from build123d import *

# Parameters (mm, degrees)
BOSS_EXTRUDE1_DEPTH = 9.5
SKETCH5_R           = 2.38125
CUT_EXTRUDE1_DEPTH  = 1.5
SKETCH9_W           = 21
SKETCH9_H           = 5
BOSS_EXTRUDE6_DEPTH = 9
SKETCH10_W          = 21
SKETCH10_H          = 14
CUT_EXTRUDE4_DEPTH  = 28.626979567
CUT_EXTRUDE5_DEPTH  = 5
SKETCH12_W          = 24
SKETCH12_H          = 9
BOSS_EXTRUDE7_DEPTH = 5
CUT_EXTRUDE6_DEPTH  = 6
SKETCH15_W          = 46
SKETCH15_H          = 3.5
CUT_EXTRUDE7_DEPTH  = 16.5
SKETCH16_W          = 12.5
SKETCH16_H          = 3.5
CUT_EXTRUDE8_DEPTH  = 16.5
BOSS_EXTRUDE8_DEPTH = 5
SKETCH18_W          = 25.5
SKETCH18_H          = 8.5
CUT_EXTRUDE9_DEPTH  = 9
BOSS_EXTRUDE9_DEPTH = 9
FILLET1_R           = 1
SKETCH20_W          = 10.25
SKETCH20_H          = 10
CUT_EXTRUDE10_DEPTH = 2
SKETCH23_W          = 1.838900381
SKETCH23_H          = 2
CUT_EXTRUDE11_DEPTH = 1.5
CHAMFER1_SIZE       = 1
CHAMFER2_SIZE       = 1


with BuildPart() as part:
    # Sketch2 → Boss-Extrude1 (new, symmetric)
    with BuildSketch(Plane.XY):
        Polygon((-12, 3), (-12, 12), (-23, 12), (-23, 0), (23, 0), (23, 12), (12, 12), (12, 3), align=None)
    extrude(amount=BOSS_EXTRUDE1_DEPTH, both=True)

    # Sketch5 → Cut-Extrude1 (cut)
    with BuildSketch(Plane(origin=(0, 12, 0), x_dir=(1, 0, 0), z_dir=(0, 1, 0))):
        with Locations(Location((-19, 1.5, 0), (0, 0, 180))):
            Circle(SKETCH5_R)
        with Locations(Location((19, 1.5, 0), (0, 0, 180))):
            Circle(SKETCH5_R)
    extrude(amount=-CUT_EXTRUDE1_DEPTH, mode=Mode.SUBTRACT)

    # Sketch9 → Boss-Extrude6 (add)
    with BuildSketch(Plane.XZ):
        with Locations((0, -7)):
            Rectangle(SKETCH9_W, SKETCH9_H)
    extrude(amount=BOSS_EXTRUDE6_DEPTH)

    # Sketch10 → Cut-Extrude4 (cut, through all)
    with BuildSketch(Plane.XZ):
        with Locations((0, 2.5)):
            Rectangle(SKETCH10_W, SKETCH10_H)
    extrude(amount=-CUT_EXTRUDE4_DEPTH, mode=Mode.SUBTRACT)

    # Sketch11 → Cut-Extrude5 (cut)
    with BuildSketch(Plane.XY.offset(9.5)):
        Polygon((10.5, 3), (10.5, 0), (23, 0), (23, 12), (12, 12), (12, 3), align=None)
        Polygon((-10.5, 0), (-10.5, 3), (-12, 3), (-12, 12), (-23, 12), (-23, 0), align=None)
    extrude(amount=-CUT_EXTRUDE5_DEPTH, mode=Mode.SUBTRACT)

    # Sketch12 → Boss-Extrude7 (add)
    with BuildSketch(Plane(origin=(0, 0, -9.5), x_dir=(-1, 0, 0), z_dir=(0, 0, -1))):
        with Locations((0, 7.5)):
            Rectangle(SKETCH12_W, SKETCH12_H)
    extrude(amount=-BOSS_EXTRUDE7_DEPTH)

    # Sketch13 → Cut-Extrude6 (cut)
    with BuildSketch(Plane.XY.offset(-4.5)):
        Polygon((-9, 12), (0, 1.274217667), (9, 12), align=None)
    extrude(amount=-CUT_EXTRUDE6_DEPTH, mode=Mode.SUBTRACT)

    # Sketch15 → Cut-Extrude7 (cut)
    with BuildSketch(Plane.XY.offset(-4.5)):
        with Locations((0, 1.75)):
            Rectangle(SKETCH15_W, SKETCH15_H)
    extrude(amount=CUT_EXTRUDE7_DEPTH, mode=Mode.SUBTRACT)

    # Sketch16 → Cut-Extrude8 (cut)
    with BuildSketch(Plane.XY.offset(-4.5)):
        with Locations((-16.75, 1.75)):
            Rectangle(SKETCH16_W, SKETCH16_H)
        with Locations((16.75, 1.75)):
            Rectangle(SKETCH16_W, SKETCH16_H)
    extrude(amount=-CUT_EXTRUDE8_DEPTH, mode=Mode.SUBTRACT)

    # Sketch17 → Boss-Extrude8 (add)
    with BuildSketch(Plane(origin=(0, 0, -9.5), x_dir=(-1, 0, 0), z_dir=(0, 0, -1))):
        Polygon((10.5, 3.5), (23, 3.5), (23, -1.5), (17, -1.5), (17, -6.5), (23, -6.709524617), (23, -9), (10.5, -9), align=None)
    extrude(amount=-BOSS_EXTRUDE8_DEPTH)

    # Sketch18 → Cut-Extrude9 (cut)
    with BuildSketch(Plane.XY.offset(-4.5)):
        with Locations((0, 7.75)):
            Rectangle(SKETCH18_W, SKETCH18_H)
    extrude(amount=CUT_EXTRUDE9_DEPTH, mode=Mode.SUBTRACT)

    # Sketch19 → Boss-Extrude9 (add)
    with BuildSketch(Plane.XY.offset(-4.5)):
        Polygon((-12.75, 3.5), (-23, 3.5), (-23, -1.5), (-17, -1.5), (-17, -6.5), (-23, -6.709524617), (-23, -9), (-12.75, -9), align=None)
    extrude(amount=BOSS_EXTRUDE9_DEPTH)

    # Fillet1
    fillet1_edges = [part.edges().sort_by_distance(p)[0] for p in [
        (-23, -1.5, -2.5),
        (-23, -6.709524617, -2.5),
    ]]
    fillet(fillet1_edges, radius=FILLET1_R)

    # Sketch20 → Cut-Extrude10 (cut)
    with BuildSketch(Plane.XY.offset(4.5)):
        with Locations((-17.875, -4)):
            Rectangle(SKETCH20_W, SKETCH20_H)
    extrude(amount=-CUT_EXTRUDE10_DEPTH, mode=Mode.SUBTRACT)

    # Sketch23 → Cut-Extrude11 (cut)
    with BuildSketch(Plane(origin=(0, 12, 0), x_dir=(1, 0, 0), z_dir=(0, 1, 0))):
        with Locations((-22.080549809, 1.5)):
            Rectangle(SKETCH23_W, SKETCH23_H)
        with Locations((22.080549809, 1.5)):
            Rectangle(SKETCH23_W, SKETCH23_H)
    extrude(amount=-CUT_EXTRUDE11_DEPTH, mode=Mode.SUBTRACT)

    # Chamfer1
    chamfer1_edges = [part.edges().sort_by_distance(p)[0] for p in [
        (-22.080549809, 12, -2.5),
        (22.080549809, 12, -2.5),
    ]]
    chamfer(chamfer1_edges, length=CHAMFER1_SIZE)

    # Chamfer2
    chamfer2_edges = [part.edges().sort_by_distance(p)[0] for p in [
        (16, 12, -9.5),
        (-16, 12, -9.5),
        (4.5, 6.637108833, -9.5),
        (-4.5, 6.637108833, -9.5),
        (23, 7.75, -9.5),
        (16.75, 3.5, -9.5),
        (-23, -8.337606696, -9.5),
        (-17, -4, -9.5),
        (-19.5, -1.5, -9.5),
        (-19.517449748, -6.587911282, -9.5),
        (-22.7193398, -6.980555021, -9.5),
        (-22.707106781, -1.207106781, -9.5),
        (10.5, -2.75, -9.5),
        (-6.25, -9, -9.5),
        (-23, 5.75, -9.5),
    ]]
    chamfer(chamfer2_edges, length=CHAMFER2_SIZE - 0.0001)  # a hair under: the kernel refuses the full size


solid = part.part
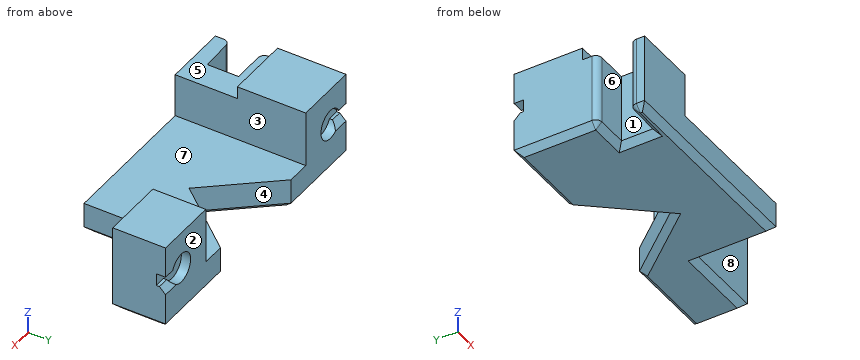
The model under review builds one solid part; all positions refer to its coordinate system, in mm. Face numbers are marked on the shaded views. A direction names the side the tool comes from. Coordinates: 2 decimals unless noted, no trailing zeros. Loops run counter-clockwise (first coordinate to the right, second up) from the corner with the lowest first, then second, coordinate; pieces in that order, holes last. Notation, with made-up numbers: (20, 43.5) -> (74, 43.5) arc R7 ccw to (74, 55.5) -> close; hole circle Ø4 at (49.5, 49.5). An arc over 180 degrees is marked (long way). Use a Markdown table: item, result. Add a question column.
1. To check wall thickness, follow line 1 (Z direction, x = -19, y = 11); line 2 (X direction, y = 11.4, z = -1.5); line 3 (X direction, y = 5.75, z = 1). State the ranges of each line that lie inside material, in increasing order.
2. Add section D-D on z = 3.5. Write out the cut boundary in (x, y), plus the area to 3 significant figures.
3. Add section A-A on z = -1.5. Write out the cut boundary in (x, y).
4. Add section B-B on x = 19. Write out the cut boundary in (y, z), plus the area to 3 significant figures.
5. Draft analysis for pull direction X (two halves, no side actions). For the marked faces 1, 2, 3 and 4, state which applies: pulls with the +X half, pulls with the -X half, needs draft (parallel to the pull), parting line crosses it, or undercut.
6. Add section C-C on y = -3. Write out the cut boundary in (x, z).
7. Machinability: for the marked faces 5, 6, 7 and 8, which of the approach directions +Z, -Z, +X, -X, +Y, -Y give a long, thin tool a straight path to every point of the face, cutting with its end or side? Answer none if there is none.
8. Clearance check with flat-ended pins moving along their axes: pin 1 Ø2.5 at (y, z) = (-5, -1.5) entering from -X; pin 2 Ø8 at (x, y) = (-15.5, -5.5) entering from +Z; pin 3 Ø1 at (x, y) = (6, 6) entering from +Z. State where each tip first meets the part, or that it passes through.
Returned:
| question | item | result |
|---|---|---|
| 1 | line 1 | z = -9.5 to -3.88, 0.88 to 4.5 |
| 1 | line 2 | x = -16.62 to -12.75, 12.75 to 16.62 |
| 1 | line 3 | x = -23 to -12.75, 12.75 to 23 |
| 2 | outline | (-23, 1) -> (-12.75, 1) -> (-12.75, 12) -> (-23, 12) -> close; (12.75, 3.5) -> (23, 3.5) -> (23, 12) -> (12.75, 12) -> close |
| 2 | area | 200 mm² |
| 3 | outline | (-23, -9) -> (-12.75, -9) -> (-12.75, 12) -> (-16.62, 12) -> (-16.62, 10.5) -> (-23, 10.5) -> (-23, -0.5) arc R1 ccw to (-22, -1.5) -> (-17, -1.5) -> (-17, -6.5) -> (-22.03, -6.68) arc R1 ccw to (-23, -7.68) -> close; (12.75, 3.5) -> (23, 3.5) -> (23, 10.5) -> (16.62, 10.5) -> (16.62, 12) -> (12.75, 12) -> close |
| 4 | outline | (3.5, -8.5) -> (4.5, -9.5) -> (11, -9.5) -> (12, -8.5) -> (12, -3.88) -> (10.5, -3.88) -> (10.5, 0.88) -> (12, 0.88) -> (12, 4.5) -> (3.5, 4.5) -> close |
| 4 | area | 111 mm² |
| 5 | face 1 | pulls with the -X half |
| 5 | face 2 | needs draft |
| 5 | face 3 | undercut |
| 5 | face 4 | undercut |
| 6 | outline | (-17, -8.5) -> (-16, -9.5) -> (9.5, -9.5) -> (10.5, -8.5) -> (10.5, -4.5) -> (-12.75, -4.5) -> (-12.75, 2.5) -> (-17, 2.5) -> close |
| 7 | face 5 | +Z, +X, -X, -Y |
| 7 | face 6 | +Z, -Z, -X |
| 7 | face 7 | +Z, +Y, -Y |
| 7 | face 8 | +Z, -Z, +X, -Y |
| 8 | pin 1 | stops at x = -17 |
| 8 | pin 2 | stops at z = 2.5 |
| 8 | pin 3 | stops at z = -4.5 |
